from build123d import *

# Parameters (mm, degrees)
F2_SIZE = 2
F3_R    = 3
F4_R    = 3


with BuildPart() as f1:
    # F0 (on Front) → F1 (revolve)
    with BuildSketch(Plane.XZ):
        Polygon((23.9498503727, 10), (-84.0501496273, 10), (-84.0501496273, -1), (-46.0501496273, -1), (-46.0501496273, -8), (-26.0501496273, -8), (-26.0501496273, -11), (-14.0501496273, -11), (-14.0501496273, -8), (-4.0501496273, -8), (-4.0501496273, 0), (0.9498503727, 0), (0.9498503727, 3), (3.9498503727, 3), (3.9498503727, 0), (8.9498503727, 0), (23.9498503727, 5), align=None)
    revolve(axis=Axis((-106.2277666089, 0, 10), (-1, 0, 0)))

    # F2
    f2_edges = [f1.edges().sort_by_distance(p)[0] for p in [
        (-84.05015, 0, 21),
        (-4.05015, 0, 28),
    ]]
    chamfer(f2_edges, length=F2_SIZE)

    # F3
    f3_edges = [f1.edges().sort_by_distance(p)[0] for p in [
        (-46.05015, 0, 28),
    ]]
    fillet(f3_edges, radius=F3_R)

    # F4
    f4_edges = [f1.edges().sort_by_distance(p)[0] for p in [
        (-46.05015, 0, 21),
    ]]
    fillet(f4_edges, radius=F4_R)


solid = f1.part
Check sheet for the modelled part. Datum: model origin and axes. Units: mm. A direction names the side the tool comes from. Give positions to 0.01 mm unless a question says otherwise; leave off trailing zeros. Order: outer loops, then holes, each group sorted by start corner. A loop starts at its lowest first (then second) coordinate and runs counter-clockwise, first axis right, second up. Notation, with made-up numbers: M 1.25,21.25 L 35.25,21.25 A13 ccw 35.25,44.25 Z; hole C 56.25,73 d10. An arc over 180 degrees is marked long. Answer as CSV lines item,"result". Start each with the question number.
Item 1: Thickness scan on line 1 (Y direction, x = -48, z = 5); line 2 (Z direction, x = 8.5, y = 0); line 3 (X direction, y = 11, z = 27). Record the ranges inside material, lowest first. Write a range as [from, to].
Item 2: Tool access check on faces 1 (the face through (0.95, 2, 17)), 2 (the face through (-34.431, -5.407, -7.169)), 3 (the face through (23.95, 0, 10)), 4 (the face through (-9.994, -5.407, -7.169)). Record the directions out of +Z, -Z, +X, -X, +Y, -Y that give a thin tool (end or side, any length) a straight path to the whole face; none if there is none.
Item 3: Gauge pin test, flat ends, axial feed: P1, Ø6, axis at x = 2, z = 11, coming from the +Y side; P2, Ø12, axis at x = -63.5, z = 0, coming from the +Y side; P3, Ø1.5, axis at x = -12, y = 14.5, coming from the -Z side. Record the tip position at first contact, or that the pin passes through.
Item 4: Cross-section at B-B on x = 12. Enter the section's corners in (y, z).
Item 5: Mould release check, pull along X, two halves, no side actions. Record for faces 5 (the face through (-65.319, 9.759, 4.924)), 6 (the face through (3.95, 2, 3)), 7 (the face through (2.471, 2.681, 3.534)), 8 (the face through (-84.05, 0, 10)): +X half, -X half, draft (parallel to the pull), parting line (faces both ways), or undercut.
Item 6: Cross-section at A-A on x = -33. Enter the section's corners in (y, z).
Established:
1,line 1,"y = [-10.01, 10.01]"
1,line 2,"z = [0, 20]"
1,line 3,"x = [-26.05, -14.05]"
2,face 1,"none"
2,face 2,"-X"
2,face 3,"+Z, -Z, +X, +Y, -Y"
2,face 4,"+X"
3,P1,"stops at y = 10"
3,P2,"stops at y = 10.25"
3,P3,"stops at z = -1.62"
4,outline,"C 0,10 d17.97"
5,face 5,"draft"
5,face 6,"undercut"
5,face 7,"undercut"
5,face 8,"-X half"
6,outline,"C 0,10 d36"
